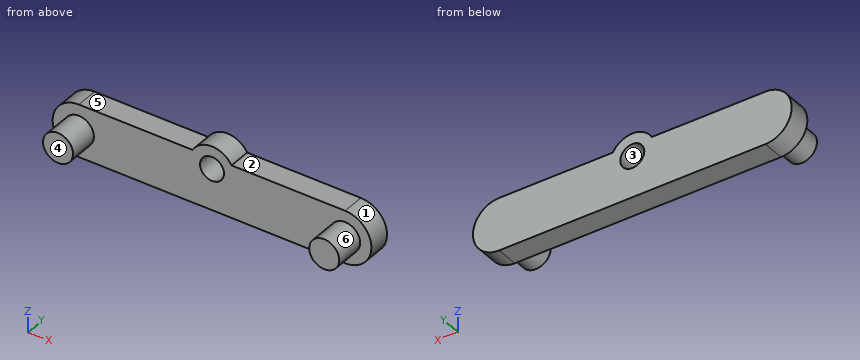
from build123d import *

# Parameters (mm, degrees)
SKETCH1_R           = 1.6
BOSS_EXTRUDE1_DEPTH = 3
SKETCH2_R           = 2
BOSS_EXTRUDE2_DEPTH = 4


with BuildPart() as part:
    # Sketch1 → Boss-Extrude1 (new body)
    with BuildSketch(Plane(origin=(0, 0, 0), x_dir=(1, 0, 0), z_dir=(0, 1, 0))):
        with BuildLine():
            Line((2.598076211, -3.5), (17.75, -3.5))
            ThreePointArc((17.75, -3.5), (21.25, 0), (17.75, 3.5))
            Line((17.75, 3.5), (-17.75, 3.5))
            ThreePointArc((-17.75, 3.5), (-21.25, 0), (-17.75, -3.5))
            Line((-17.75, -3.5), (-2.598076211, -3.5))
            ThreePointArc((-2.598076211, -3.5), (0, -5), (2.598076211, -3.5))
        make_face()
        with Locations(Location((0, -2, 0), (0, 0, 270))):
            Circle(SKETCH1_R, mode=Mode.SUBTRACT)
    extrude(amount=BOSS_EXTRUDE1_DEPTH)

    # Sketch2 → Boss-Extrude2 (add)
    with BuildSketch(Plane.XZ):
        with Locations(Location((-17.75, 0, 0), (0, 0, 90))):
            Circle(SKETCH2_R)
        with Locations(Location((17.75, 0, 0), (0, 0, 90))):
            Circle(SKETCH2_R)
    extrude(amount=BOSS_EXTRUDE2_DEPTH)


solid = part.part
Design review of the part built by this model. Coordinates are the model's own, in mm. Face numbers are marked on the shaded views. A direction names the side the tool comes from. Give positions to 0.01 mm unless a question says otherwise; leave off trailing zeros. Order: outer loops, then holes, each group sorted by start corner. A loop starts at its lowest first (then second) coordinate and runs counter-clockwise, first axis right, second up. Notation, with made-up numbers: (-37.75, 28.25) - (-26.75, 28.25) arc R33 cw to (-26.75, 63.25) - close; hole circle Ø9 at (-10, 68.25). An arc over 180 degrees is marked (long way). Write item = value, one per line. Start each with the question number.
Q1. To check wall thickness, follow L1, parallel to Z at x = 12, y = 2; L2, parallel to Y at x = 7, z = 0; L3, parallel to X at y = 1.25, z = 2. State the ranges of each line that lie inside material, in increasing order. Write a range as from..to.
Q2. We need section B-B on y = 1.75. State the section outline as (x, z) points, plus the area to 3 significant figures.
Q3. We need section D-D on y = -1.5. State the section outline as (x, z) points, plus the area to 3 significant figures.
Q4. Mouldability with a two-part tool opening along Z and no side actions: class the marked faces 1, 2 and 3 as released by +Z, released by -Z, zero draft, split by the parting line, or undercut.
Q5. Clearance check with flat-ended pins moving along their axes: pin 1 Ø3 at (x, y) = (2, 2) entering from +Z; pin 2 Ø3.5 at (x, z) = (0, 2) entering from -Y; pin 3 Ø0.9 at (x, y) = (13.5, 2) entering from +Z. State where each tip first meets the part, or that it passes through.
Q6. We need section C-C on z = 1.25. State the section outline as (x, y) points.
Q7. We need section A-A on x = 0. State the section outline as (y, z) points, plus the area to 3 significant figures.
Q8. Tool access review of the marked faces 4, 5 and 6: name each direction out of +Z, -Z, +X, -X, +Y, -Y from which nothing blocks a thin tool from reaching the whole face with its end or side.
Working result:
q1.L1 = -3.5..3.5
q1.L2 = 0..3
q1.L3 = -20.62..-1.6, 1.6..20.62
q2.outline = (-17.75, -3.5) - (17.75, -3.5) arc R3.5 ccw to (17.75, 3.5) - (2.6, 3.5) arc R3 ccw to (-2.6, 3.5) - (-17.75, 3.5) arc R3.5 ccw to start; hole circle Ø3.2 at (0, 2)
q2.area = 284 mm²
q3.outline = circle Ø4 at (-17.75, 0); circle Ø4 at (17.75, 0)
q3.area = 25.1 mm²
q4.face_1 = split by the parting line
q4.face_2 = released by +Z
q4.face_3 = undercut
q5.pin_1 = 4.96
q5.pin_2 = 0
q5.pin_3 = 3.5
q6.outline = (-21.02, 0) - (-19.31, 0) - (-19.31, -4) - (-16.19, -4) - (-16.19, 0) - (-1.41, 0) - (-1.41, 3) - (-21.02, 3) - close; (1.41, 0) - (16.19, 0) - (16.19, -4) - (19.31, -4) - (19.31, 0) - (21.02, 0) - (21.02, 3) - (1.41, 3) - close
q7.outline = (0, -3.5) - (3, -3.5) - (3, 0.4) - (0, 0.4) - close; (0, 3.6) - (3, 3.6) - (3, 5) - (0, 5) - close
q7.area = 15.9 mm²
q8.face_4 = +Z, -Z, +X, -X, -Y
q8.face_5 = +Z, -X, +Y, -Y
q8.face_6 = -Y
